Could you check a few things on this model? Use its own coordinates, in mm. Face numbers are marked on the shaded views. Coordinates: 2 decimals unless noted, no trailing zeros. Write each loop counter-clockwise with the first axis right and the second up, starting at its lowest first coordinate (ties: lowest second). Pieces come first, ordered by that corner, then holes. Notation, with made-up numbers: (83, 5.25) - (142, 5.25) arc R21 ccw to (142, 31.25) - close; hole circle Ø10 at (39, 0). An arc over 180 degrees is marked (long way). Answer as a JSON object with one key per item and string values. Group by question number.
1) If we section it at C-C (x = -20): Write out the boundary of the cut face in (y, z).
2) If we section it at D-D (x = 6.5): Write out the boundary of the cut face in (y, z), plus the area to 3 significant figures.
3) If we section it at B-B (z = 5.5): Write out the boundary of the cut face in (x, y).
4) If we section it at A-A (x = -2.5): Write out the boundary of the cut face in (y, z).
5) We'd pull the mould along Z, two halves only. Please class the marked faces 1 and 2: released by +Z, released by -Z, zero draft, split by the parting line, or undercut.
6) Please list where these lines run through material, in increasing order: line 1 along X through (y, z) = (3.75, -8.5); line 2 along Z through (x, y) = (5, 1.25); line 3 along Z through (x, y) = (11, 4.5).
7) Will these pins go through, and if not, where does the flat tip stop? pin 1 Ø1.6 at (y, z) = (4, -8.5) entering from +X; pin 2 Ø0.6 at (x, z) = (8.5, -1.5) entering from +Y; pin 3 Ø3 at (x, z) = (24.5, -17.5) entering from +Y.
```python
from build123d import *

# Parameters (mm, degrees)
BOSS_EXTRUDE1_DEPTH = 2
SKETCH1_3_W         = 62.50000000000001
SKETCH1_3_H         = 92.5
BOSS_EXTRUDE2_DEPTH = 6
BOSS_EXTRUDE3_DEPTH = 6
CUT_EXTRUDE2_DEPTH  = 39.00000000000001
CUT_EXTRUDE3_START  = 2
CUT_EXTRUDE3_DEPTH  = 8
FILLET1_R           = 4
BOSS_EXTRUDE4_DEPTH = 1
CUT_EXTRUDE7_DEPTH  = 4
FILLET2_R           = 3
SKETCH9_W           = 5.999999999999999
SKETCH9_H           = 6
SKETCH9_H_2         = 5.999999999999999
CUT_EXTRUDE8_DEPTH  = 10


with BuildPart() as part:
    # Sketch1 → Boss-Extrude1 (new body)
    with BuildSketch(Plane(origin=(0, 0, 0), x_dir=(1, 0, 0), z_dir=(0, 1, 0))):
        Polygon((-32.5, 47.74999999999999), (32.5, 47.74999999999999), (32.50000000000001, -47.75000000000001), (-32.49999999999998, -47.75000000000001), align=None)
    extrude(amount=BOSS_EXTRUDE1_DEPTH)

    # Sketch1<3> → Boss-Extrude2 (add)
    with BuildSketch(Plane(origin=(0, 0, 0), x_dir=(1, 0, 0), z_dir=(0, 1, 0))):
        Rectangle(SKETCH1_3_W, SKETCH1_3_H)
    extrude(amount=BOSS_EXTRUDE2_DEPTH)

    # Sketch2<4> → Boss-Extrude3 (add)
    with BuildSketch(Plane(origin=(0, 0, 0), x_dir=(1, 0, 0), z_dir=(0, 1, 0))):
        Polygon((-9.799999999999999, -9.799999999999999), (9.799999999999999, -9.799999999999999), (9.799999999999997, 9.799999999999999), (-9.8, 9.799999999999999), align=None)
    extrude(amount=BOSS_EXTRUDE3_DEPTH)

    # Sketch2 → Cut-Extrude2 (cut)
    with BuildSketch(Plane(origin=(0, 0, 0), x_dir=(1, 0, 0), z_dir=(0, 1, 0))):
        with BuildLine():
            Line((-7.800000000000002, 7.800000000000001), (-7.8, -7.799999999999999))
            Line((-7.8, -7.799999999999999), (7.8, -7.799999999999999))
            Line((7.8, -7.799999999999999), (7.8, -0.7999999999999989))
            ThreePointArc((7.8, -0.7999999999999985), (8.928220211291862, 1.0000000000000016), (7.799999999999999, 2.8000000000000007))
            Line((7.7999999999999785, 2.8000000000000007), (7.799999999999998, 7.800000000000001))
            Line((7.799999999999998, 7.800000000000001), (-7.800000000000002, 7.800000000000001))
        make_face()
    extrude(amount=CUT_EXTRUDE2_DEPTH, mode=Mode.SUBTRACT)

    # Sketch3 → Cut-Extrude3 (cut)
    with BuildSketch(Plane(origin=(0, 0, 0), x_dir=(1, 0, 0), z_dir=(0, 1, 0)).offset(CUT_EXTRUDE3_START)):
        with BuildLine():
            Line((-30.43328770425558, 49.15666281909306), (-34.56671229574442, 46.343337180906936))
            Line((-34.56671229574442, 46.343337180906936), (-30.34672383846524, 40.14320029367368))
            ThreePointArc((-30.346723838465234, 40.14320029367369), (-26.87334872362776, 39.48315081702232), (-26.213299246976405, 42.9565259318598))
            Line((-26.2132992469764, 42.9565259318598), (-30.43328770425558, 49.15666281909306))
        make_face()
        with BuildLine():
            Line((34.56671229574442, 46.343337180906936), (30.43328770425558, 49.15666281909306))
            Line((30.43328770425558, 49.15666281909306), (26.21329924697641, 42.9565259318598))
            ThreePointArc((26.213299246976415, 42.956525931859794), (26.87334872362777, 39.48315081702232), (30.346723838465245, 40.14320029367368))
            Line((30.346723838465245, 40.14320029367368), (34.56671229574442, 46.343337180906936))
        make_face()
        with BuildLine():
            Line((-30.346723838465223, -40.143200293673694), (-34.566712295744395, -46.34333718090695))
            Line((-34.566712295744395, -46.34333718090695), (-30.43328770425555, -49.15666281909307))
            Line((-30.43328770425555, -49.15666281909307), (-26.213299246976373, -42.95652593185982))
            ThreePointArc((-26.213299246976383, -42.956525931859815), (-26.873348723627743, -39.48315081702233), (-30.346723838465227, -40.143200293673694))
        make_face()
        with BuildLine():
            Line((26.213299246976398, -42.95652593185982), (30.433287704255594, -49.15666281909309))
            Line((30.433287704255594, -49.15666281909309), (34.56671229574444, -46.34333718090698))
            Line((34.56671229574444, -46.34333718090698), (30.34672383846524, -40.143200293673694))
            ThreePointArc((30.346723838465252, -40.14320029367369), (26.873348723627778, -39.48315081702233), (26.213299246976423, -42.95652593185981))
        make_face()
    extrude(amount=CUT_EXTRUDE3_DEPTH, mode=Mode.SUBTRACT)

    # Fillet1
    # the kernel refuses this fillet: 4 mm, written as the material it takes off along each edge
    with BuildSketch(Plane(origin=(-36.87665127637225, 6, 49.73717060629096), x_dir=(-0.8266849182977679, 0, -0.5626651276372232), z_dir=(0.5626651276372232, 0, -0.826684918297768))) as fillet1_piece_1:
        with BuildLine():
            CenterArc((FILLET1_R, -FILLET1_R), FILLET1_R, 90, 90)
            Line((0, -FILLET1_R), (0, 0))
            Line((0, 0), (FILLET1_R, 0))
        make_face()
    extrude(amount=11.605353019348973, mode=Mode.SUBTRACT)
    with BuildSketch(Plane(origin=(-26.213299246976373, 6, 42.95652593185982), x_dir=(0.8266849182977672, 0, 0.5626651276372243), z_dir=(-0.5626651276372243, 0, 0.8266849182977672))) as fillet1_piece_2:
        with BuildLine():
            CenterArc((FILLET1_R, -FILLET1_R), FILLET1_R, 90, 90)
            Line((-1.06e-15, -FILLET1_R), (0, 0))
            Line((0, 0), (FILLET1_R, 0))
        make_face()
    extrude(amount=13.983953251405376, mode=Mode.SUBTRACT)
    with BuildSketch(Plane(origin=(34.0815820880514, 6, 54.51684918297768), x_dir=(-0.826684918297767, 0, 0.5626651276372246), z_dir=(-0.5626651276372246, 0, -0.826684918297767))) as fillet1_piece_3:
        with BuildLine():
            CenterArc((FILLET1_R, -FILLET1_R), FILLET1_R, 90, 90)
            Line((-1.88e-15, -FILLET1_R), (0, 0))
            Line((0, 0), (FILLET1_R, 0))
        make_face()
    extrude(amount=13.983953251405392, mode=Mode.SUBTRACT)
    with BuildSketch(Plane(origin=(30.346723838465245, 6, 40.1432002936737), x_dir=(0.8266849182977677, 0, -0.5626651276372238), z_dir=(0.5626651276372238, 0, 0.8266849182977677))) as fillet1_piece_4:
        with BuildLine():
            CenterArc((FILLET1_R, -FILLET1_R), FILLET1_R, 90, 90)
            Line((0, -FILLET1_R), (0, 0))
            Line((0, 0), (FILLET1_R, 0))
        make_face()
    extrude(amount=11.605353019348959, mode=Mode.SUBTRACT)
    with BuildSketch(Plane(origin=(36.87665127637224, 6, -49.73717060629088), x_dir=(0.8266849182977675, 0, 0.562665127637224), z_dir=(-0.562665127637224, 0, 0.8266849182977676))) as fillet1_piece_5:
        with BuildLine():
            CenterArc((FILLET1_R, -FILLET1_R), FILLET1_R, 90, 90)
            Line((-4e-15, -FILLET1_R), (0, 0))
            Line((0, 0), (FILLET1_R, 0))
        make_face()
    extrude(amount=11.605353019348904, mode=Mode.SUBTRACT)
    with BuildSketch(Plane(origin=(26.21329924697641, 6, -42.9565259318598), x_dir=(-0.826684918297768, 0, -0.5626651276372232), z_dir=(0.5626651276372232, 0, -0.826684918297768))) as fillet1_piece_6:
        with BuildLine():
            CenterArc((FILLET1_R, -FILLET1_R), FILLET1_R, 90, 90)
            Line((-1.88e-15, -FILLET1_R), (0, 0))
            Line((0, 0), (FILLET1_R, 0))
        make_face()
    extrude(amount=13.98395325140539, mode=Mode.SUBTRACT)
    with BuildSketch(Plane(origin=(-34.08158208805138, 6, -54.51684918297765), x_dir=(0.8266849182977676, 0, -0.562665127637224), z_dir=(0.562665127637224, 0, 0.8266849182977676))) as fillet1_piece_7:
        with BuildLine():
            CenterArc((FILLET1_R, -FILLET1_R), FILLET1_R, 90, 90)
            Line((0, -FILLET1_R), (0, 0))
            Line((0, 0), (FILLET1_R, 0))
        make_face()
    extrude(amount=13.983953251405376, mode=Mode.SUBTRACT)
    with BuildSketch(Plane(origin=(-30.34672383846524, 6, -40.14320029367368), x_dir=(-0.8266849182977674, 0, 0.5626651276372242), z_dir=(-0.5626651276372242, 0, -0.8266849182977674))) as fillet1_piece_8:
        with BuildLine():
            CenterArc((FILLET1_R, -FILLET1_R), FILLET1_R, 90, 90)
            Line((1.06e-15, -FILLET1_R), (0, 0))
            Line((0, 0), (FILLET1_R, 0))
        make_face()
    extrude(amount=11.605353019348907, mode=Mode.SUBTRACT)
    with BuildSketch(Plane(origin=(-28.2800115427208, 6, 41.549863112766744), x_dir=(-0.8266849182977704, 0, -0.5626651276372198), z_dir=(-0.5626651276372198, 0, 0.8266849182977704))) as fillet1_piece_9:
        with BuildLine():
            CenterArc((2.5000000000000013 + FILLET1_R, FILLET1_R), FILLET1_R, 180, 90)
            Line((2.4999999999999996, FILLET1_R), (2.5000000000000013, 0))
            Line((2.5000000000000013, 0), (2.5000000000000013 + FILLET1_R, 0))
        make_face()
    revolve(axis=Axis((-28.2800115427208, 6, 41.549863112766744), (0, -1, 0)), revolution_arc=180.0000000000006, mode=Mode.SUBTRACT)
    with BuildSketch(Plane(origin=(28.280011542720835, 6, 41.549863112766744), x_dir=(-0.8266849182977659, 0, 0.5626651276372262), z_dir=(0.5626651276372262, 0, 0.8266849182977659))) as fillet1_piece_10:
        with BuildLine():
            CenterArc((2.499999999999998 + FILLET1_R, FILLET1_R), FILLET1_R, 180, 90)
            Line((2.4999999999999996, FILLET1_R), (2.499999999999998, 0))
            Line((2.499999999999998, 0), (2.499999999999998 + FILLET1_R, 0))
        make_face()
    revolve(axis=Axis((28.280011542720835, 6, 41.549863112766744), (0, -1, 0)), revolution_arc=180.00000000000017, mode=Mode.SUBTRACT)
    with BuildSketch(Plane(origin=(28.28001154272083, 6, -41.54986311276673), x_dir=(0.826684918297769, 0, 0.5626651276372218), z_dir=(0.5626651276372218, 0, -0.826684918297769))) as fillet1_piece_11:
        with BuildLine():
            CenterArc((2.499999999999993 + FILLET1_R, FILLET1_R), FILLET1_R, 180, 90)
            Line((2.49999999999999, FILLET1_R), (2.499999999999993, 0))
            Line((2.499999999999993, 0), (2.499999999999993 + FILLET1_R, 0))
        make_face()
    revolve(axis=Axis((28.28001154272083, 6, -41.54986311276673), (0, -1, 0)), revolution_arc=180.00000000000037, mode=Mode.SUBTRACT)
    with BuildSketch(Plane(origin=(-28.280011542720814, 6, -41.54986311276674), x_dir=(0.8266849182977655, 0, -0.562665127637227), z_dir=(-0.562665127637227, 0, -0.8266849182977655))) as fillet1_piece_12:
        with BuildLine():
            CenterArc((2.499999999999995 + FILLET1_R, FILLET1_R), FILLET1_R, 180, 90)
            Line((2.499999999999995, FILLET1_R), (2.499999999999995, 0))
            Line((2.499999999999995, 0), (2.499999999999995 + FILLET1_R, 0))
        make_face()
    revolve(axis=Axis((-28.280011542720814, 6, -41.54986311276674), (0, -1, 0)), revolution_arc=180.0000000000004, mode=Mode.SUBTRACT)

    # Sketch7 → Boss-Extrude4 (add)
    with BuildSketch(Plane(origin=(0, 0, 0), x_dir=(1, 0, 0), z_dir=(0, 1, 0))):
        with BuildLine():
            Line((7.799999999999999, 2.8000000000000003), (7.799999999999998, -0.799999999999999))
            ThreePointArc((7.799999999999998, -0.799999999999999), (8.928220211291862, 1.0000000000000004), (7.799999999999999, 2.8000000000000003))
        make_face()
    extrude(amount=BOSS_EXTRUDE4_DEPTH)

    # Sketch5 → Cut-Extrude7 (cut)
    with BuildSketch(Plane(origin=(0, 6, 0), x_dir=(1, 0, 0), z_dir=(0, 1, 0))):
        Polygon((-21.75628660862557, -45.25000000000001), (21.756286608625608, -45.25000000000001), (30.25, -45.25000000000001), (30.25, -34.31321019320602), (30.25, 34.31321019320601), (30.25, 45.24999999999999), (21.7562866086256, 45.24999999999999), (-21.75628660862558, 45.24999999999999), (-30.25, 45.24999999999999), (-30.25, 34.31321019320601), (-30.25, -34.31321019320603), (-30.25, -45.25000000000001), align=None)
        Polygon((9.799999999999999, -9.799999999999999), (-9.799999999999999, -9.799999999999999), (-9.800000000000002, 9.799999999999999), (9.799999999999995, 9.799999999999999), align=None, mode=Mode.SUBTRACT)
    extrude(amount=-CUT_EXTRUDE7_DEPTH, mode=Mode.SUBTRACT)

    # Fillet2
    fillet2_edges = [part.edges().sort_by_distance(p)[0] for p in [
        (-32.5, 1, -47.74999999999999),
        (32.5, 1, -47.74999999999999),
        (32.50000000000001, 1, 47.75000000000001),
        (-32.49999999999998, 1, 47.75000000000001),
    ]]
    fillet(fillet2_edges, radius=FILLET2_R)

    # Sketch9 → Cut-Extrude8 (cut)
    with BuildSketch(Plane(origin=(0, 2, 0), x_dir=(1, 0, 0), z_dir=(0, 1, 0))):
        Polygon((-9.800000000000002, 9.799999999999999), (-3.800000000000001, 9.799999999999999), (-3.8000000000000003, 3.7999999999999994), (-9.800000000000002, 3.7999999999999994), align=None)
        with Locations((-6.799999999999999, -6.799999999999999)):
            Rectangle(SKETCH9_W, SKETCH9_H)
        with Locations((6.799999999999999, -6.799999999999999)):
            Rectangle(SKETCH9_W, SKETCH9_H_2)
        Polygon((9.799999999999995, 9.799999999999999), (3.7999999999999954, 9.799999999999999), (3.7999999999999963, 3.7999999999999985), (9.799999999999995, 3.7999999999999994), align=None)
    extrude(amount=CUT_EXTRUDE8_DEPTH, mode=Mode.SUBTRACT)


solid = part.part
```
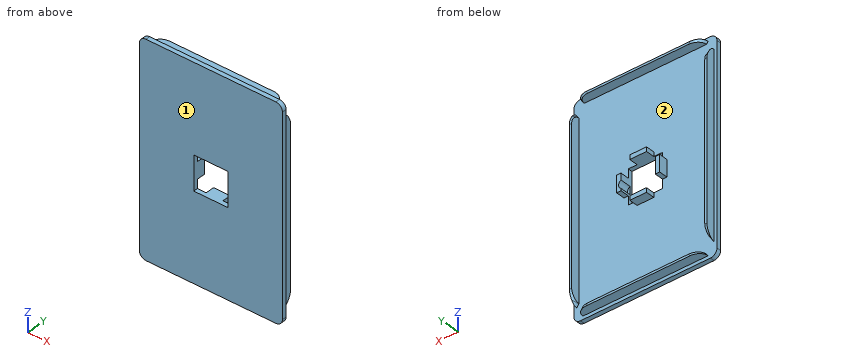
Here are the results:
{
 "1": {"outline": "(0, -47.75) - (2, -47.75) - (2, -46.25) - (6, -46.25) - (6, -45.25) - (2, -45.25) - (2, 45.25) - (6, 45.25) - (6, 46.25) - (2, 46.25) - (2, 47.75) - (0, 47.75) - close"},
 "2": {"outline": "(0, -47.75) - (2, -47.75) - (2, -46.25) - (6, -46.25) - (6, -45.25) - (2, -45.25) - (2, -7.8) - (0, -7.8) - close; (0, 7.8) - (2, 7.8) - (2, 45.25) - (6, 45.25) - (6, 46.25) - (2, 46.25) - (2, 47.75) - (0, 47.75) - close", "area": "168 mm²"},
 "3": {"outline": "(-32.5, 0) - (-7.8, 0) - (-7.8, 2) - (-30.25, 2) - (-30.25, 6) - (-31.25, 6) - (-31.25, 2) - (-32.5, 2) - close; (7.8, 0) - (32.5, 0) - (32.5, 2) - (31.25, 2) - (31.25, 6) - (30.25, 6) - (30.25, 2) - (7.8, 2) - close"},
 "4": {"outline": "(0, -47.75) - (2, -47.75) - (2, -46.25) - (6, -46.25) - (6, -45.25) - (2, -45.25) - (2, -9.8) - (6, -9.8) - (6, -7.8) - (0, -7.8) - close; (0, 7.8) - (6, 7.8) - (6, 9.8) - (2, 9.8) - (2, 45.25) - (6, 45.25) - (6, 46.25) - (2, 46.25) - (2, 47.75) - (0, 47.75) - close"},
 "5": {"face 1": "zero draft", "face 2": "undercut"},
 "6": {"line 1": "x = -31.25 to -30.25, -3.8 to 3.8, 30.25 to 31.25", "line 2": "z = -47.75 to -7.8, 7.8 to 47.75", "line 3": "z = -46.25 to -45.25, 45.25 to 46.25"},
 "7": {"pin 1": "stops at x = 31.25", "pin 2": "stops at y = 1", "pin 3": "stops at y = 2"}
}
